Design review of the part built by this model. Coordinates are the model's own, in mm. Face numbers are marked on the shaded views. A direction names the side the tool comes from. Give positions to 0.01 mm unless a question says otherwise; leave off trailing zeros. Return JSON: item names as keys, results as strings. Group by question number.
from build123d import *

# Parameters (mm, degrees)
TAP_DRILL_FOR_M7X1_0_TAP3_D     = 6
TAP_DRILL_FOR_M7X1_0_TAP3_DEPTH = 10.5


with BuildPart() as part:
    # Sketch1 → Revolve1 (revolve)
    with BuildSketch(Plane.XY):
        Polygon((0, 0), (-8, 0), (-8, -3.7), (-6, -3.7), (-6, -9.7), (-8, -9.7), (-8, -12.7), (-4.5, -12.7), (-4.5, -14.2), (-8, -14.2), (-8, -15.2), (-4.659090909, -15.2), (-4.659090909, -16.7), (-11.15, -16.7), (-11.15, -17.7), (-4.818181818, -17.7), (-4.818181818, -19.2), (-11.15, -19.2), (-11.15, -20.2), (-4.977272727, -20.2), (-4.977272727, -21.7), (-11.15, -21.7), (-11.15, -22.7), (-5.136363636, -22.7), (-5.136363636, -24.2), (-11.15, -24.2), (-11.15, -25.2), (-5.295454545, -25.2), (-5.295454545, -26.7), (-11.15, -26.7), (-11.15, -27.7), (-5.454545455, -27.7), (-5.454545455, -29.2), (-11.15, -29.2), (-11.15, -30.2), (-5.613636364, -30.2), (-5.613636364, -31.7), (-11.15, -31.7), (-11.15, -32.7), (-5.772727273, -32.7), (-5.772727273, -34.2), (-11.15, -34.2), (-11.15, -35.2), (-5.931818182, -35.2), (-5.931818182, -36.7), (-11.15, -36.7), (-11.15, -37.7), (-6.090909091, -37.7), (-6.090909091, -39.2), (-11.15, -39.2), (-11.15, -40.2), (-6.25, -40.2), (-6.25, -41.7), (-11.15, -41.7), (-11.15, -42.7), (0, -42.7), align=None)
    revolve(axis=Axis((0, -42.7, 0), (0, 1, 0)))

    # Tap Drill for M7x1.0 Tap3
    with Locations(Plane(origin=(0, -42.7, 0), x_dir=(-1, 0, 0), z_dir=(0, -1, 0))):
        with Locations((0, 0)):
            Hole(TAP_DRILL_FOR_M7X1_0_TAP3_D / 2, depth=TAP_DRILL_FOR_M7X1_0_TAP3_DEPTH)

    # Sketch1<4> → Cut-Revolve1 (revolve, cut)
    with BuildSketch(Plane.XY):
        Polygon((0, -42.7), (0, 0), (-4, 0), (-4, -6.5), (-2, -7.654700538), (-2, -27.29955572), (-2, -42.7), align=None)
    revolve(axis=Axis((0, -42.7, 0), (0, 1, 0)), mode=Mode.SUBTRACT)


solid = part.part
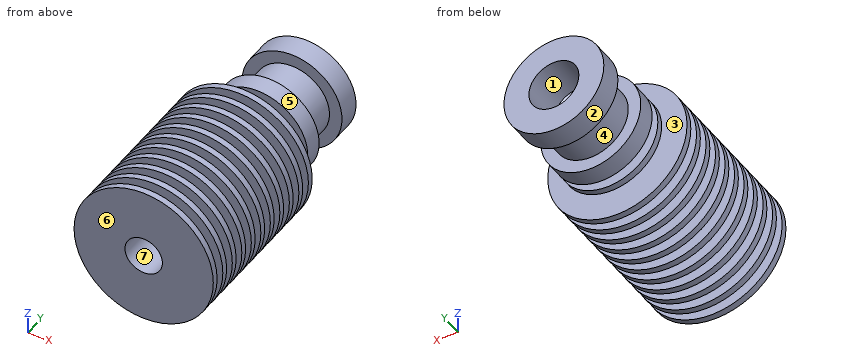
Q1. Take a section at A-A, the plane x = -6.75. Count the separate pieces of the cut face and the enclosed holes in it, plus the area to 3 significant figures.
Q2. Tool access review of the marked faces 4, 5, 6 and 7: name each direction out of +Z, -Z, +X, -X, +Y, -Y from which nothing blocks a thin tool from reaching the whole face with its end or side.
Q3. Mouldability with a two-part tool opening along Z and no side actions: class the marked faces 1, 2 and 3 as +Z half, -Z half, draft (parallel to the pull), parting line (faces both ways), or undercut.
Q4. For L1, parallel to Z at x = 0, y = -34.5; L2, parallel to Z at x = 0, y = -22.75; L3, parallel to X at y = -6, z = -0.25, list the stretches that pass through material, from the lowest coordinate up. Write a range as from..to.
Q5. Insertion check: pin 1 (4 mm diameter, centred on x = -7, y = -19.5, fed in from -Z); pin 2 (1 mm diameter, centred on y = -15.5, z = 4.5, fed in from +X); pin 3 (12 mm diameter, centred on y = -14, z = 5.5, fed in from -X); pin 4 (6.5 mm diameter, centred on x = 0.5, z = 1, fed in from +Y). Each pin has a flat end and moves straight along its axis. Give the tip position at first contact, or say it passes through.
Final values:
{
 "1": {"separate pieces": "14", "enclosed holes": "0", "area": "261 mm²"},
 "2": {"face 4": "none", "face 5": "+Y", "face 6": "+Z, -Z, +X, -X, -Y", "face 7": "-Y"},
 "3": {"face 1": "undercut", "face 2": "parting line", "face 3": "draft"},
 "4": {"L1": "z = -11.15..-3, 3..11.15", "L2": "z = -5.14..-2, 2..5.14", "L3": "x = -5.99..-3.99, 3.99..5.99"},
 "5": {"pin 1": "stops at z = -9.97", "pin 2": "stops at x = 6.87", "pin 3": "stops at x = -11.15", "pin 4": "stops at y = 0"}
}
